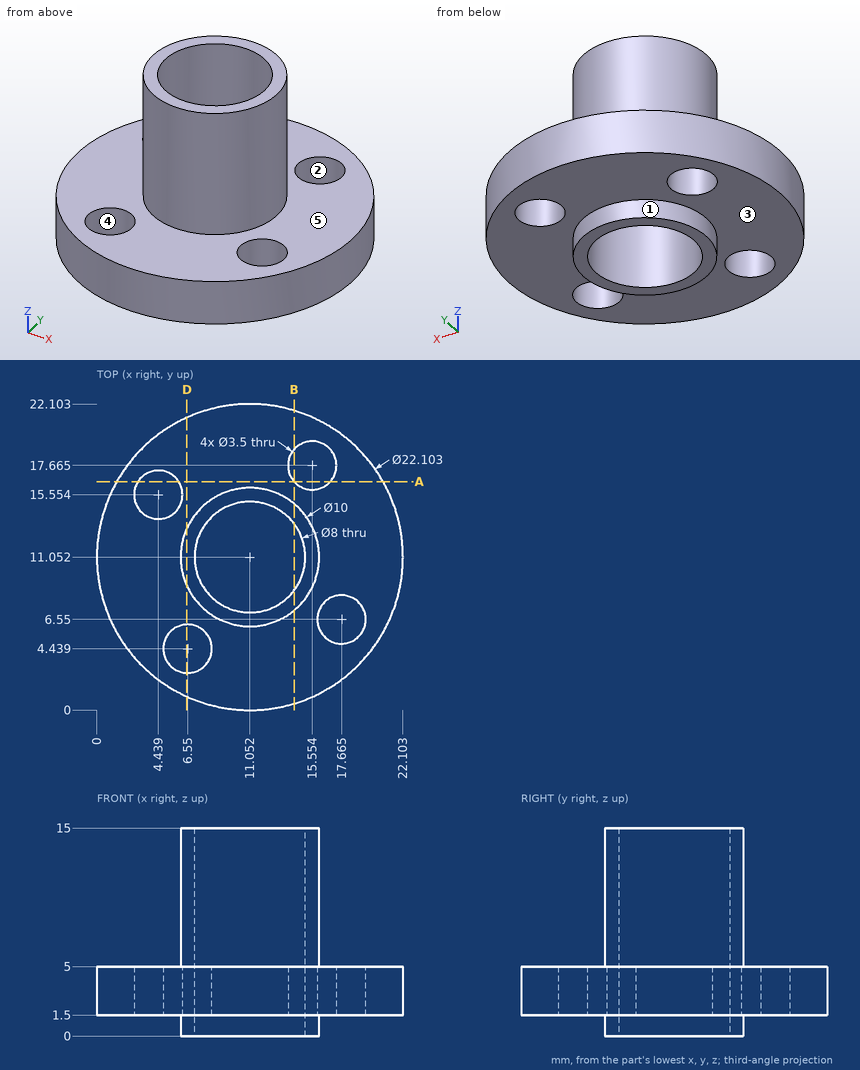
Job drawing, mm, ordinate dimensions from the low corner. One solid piece. A direction names the side the tool comes from. Coordinates: 2 decimals unless noted, no trailing zeros. Write each loop counter-clockwise with the first axis right and the second up, starting at its lowest first coordinate (ties: lowest second). Pieces come first, ordered by that corner, then holes.
Item 1: Slice it at D-D (x = 6.5). Write the cut outline in (y, z), and give its area (3 significant figures).
Item 2: Probe line 1 (X direction, y = 11.25, z = 4.5); line 2 (X direction, y = 5.25, z = 2.25) (1 decimal). List the from-to ranges inside material, lowest first.
Item 3: Slice it at B-B (x = 14.25). Count the separate pieces of the cut face and the enclosed holes in it.
Item 4: Slice it at A-A (y = 16.5). Write the cut outline in (x, z).
Item 5: Which spindle directions (+Z, -Z, +X, -X, +Y, -Y) get a long thin tool onto all of the face, cutting with end or side? Do the marked faces 4 and 5. Say none if no direction does.
Item 6: Pin check, flat tips, straight feed: pin 1 (1.5 mm diameter, centred on y = 3.5, z = 10, fed in from +X); pin 2 (1.5 mm diameter, centred on y = 12, z = 11, fed in from +X); pin 3 (3 mm diameter, centred on x = 16, z = 7, fed in from -Y); pin 4 (4 mm diameter, centred on x = 6.55, y = 4.44, fed in from +Z). Stop position of each tip, or through.
Item 7: Mould opens along X. For the marked faces 1, 2 and 3 say: released by +X, released by -X, zero draft, split by the parting line, or undercut.
Results found:
1. outline: (0.98, 1.5) - (2.69, 1.5) - (2.69, 5) - (0.98, 5) - close; (6.19, 1.5) - (8.98, 1.5) - (8.98, 0) - (13.12, 0) - (13.12, 1.5) - (21.12, 1.5) - (21.12, 5) - (13.12, 5) - (13.12, 15) - (8.98, 15) - (8.98, 5) - (6.19, 5) - close
1. area: 106 mm2
2. line 1: x = 0 to 7.06, 15.05 to 22.1
2. line 2: x = 1.6 to 5, 8.1 to 16.5, 18.8 to 20.5
3. separate pieces: 3
3. enclosed holes: 0
4. outline: (1.44, 1.5) - (2.97, 1.5) - (2.97, 5) - (1.44, 5) - close; (5.91, 1.5) - (14.25, 1.5) - (14.25, 5) - (5.91, 5) - close; (16.86, 1.5) - (20.67, 1.5) - (20.67, 5) - (16.86, 5) - close
5. face 4: +Z, -Z
5. face 5: +Z
6. pin 1: passes through
6. pin 2: stops at x = 16.05
6. pin 3: stops at y = 7.43
6. pin 4: stops at z = 5
7. face 1: split by the parting line
7. face 2: undercut
7. face 3: zero draft
